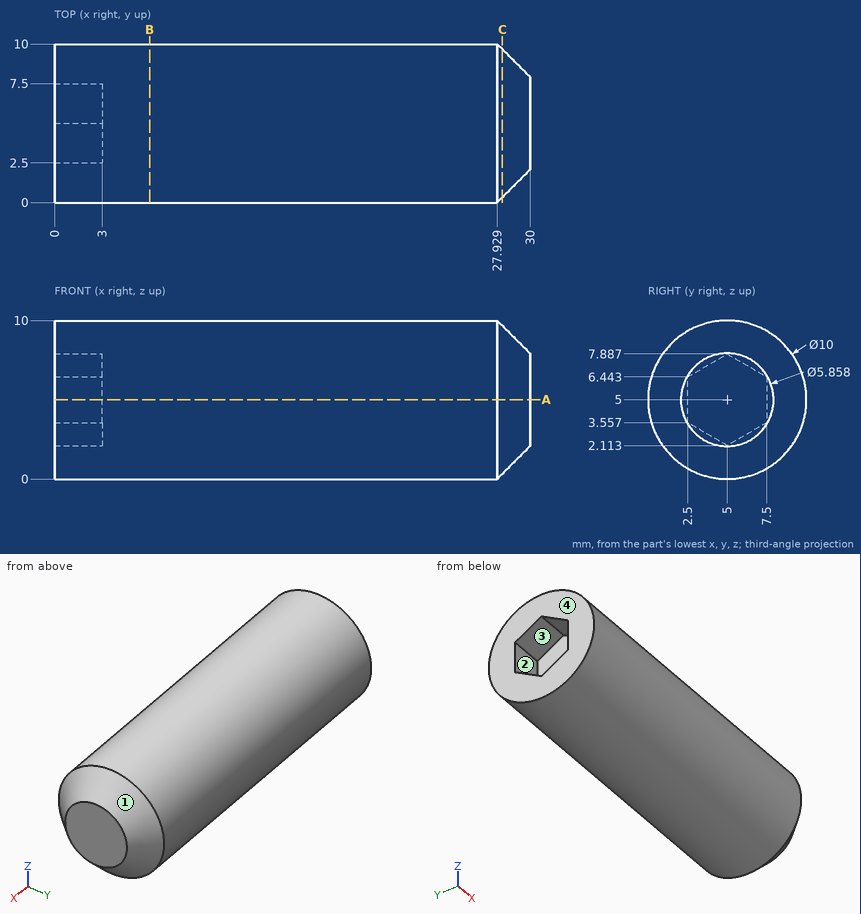
Study the drawing (mm; zero at the part's minimum x, y, z) and answer. Coordinates: 2 decimals unless noted, no trailing zeros. Order: outer loops, then holes, each group sorted by start corner. A loop starts at its lowest first (then second) coordinate and runs counter-clockwise, first axis right, second up. Notation, with made-up numbers: (81.25, -19.5) -> (90.25, -19.5) arc R19 cw to (90.25, 10.5) -> close; hole circle Ø6 at (-0.5, 79.5). An arc over 180 degrees is marked (long way). Answer in a Markdown table with one row per item. Add a question column.
Item 1: Find the intervals of material crossed by L1, parallel to Z at x = 9.25, y = 5.25; L2, parallel to X at y = 4.25, z = 5.5; L3, parallel to Y at x = 2.25, z = 4.5 (1 decimal), in increasing order. Write a range as from..to.
Item 2: Find section A-A (z = 5). Write down the section's boundary in (x, y).
Item 3: Each of these flat-tipped pins is pushed along its axis until it touches: P1, Ø3, axis at x = 23.5, z = 7, coming from the -Y side (1 decimal); P2, Ø3, axis at x = 21, y = 2.5, coming from the -Z side; P3, Ø1, axis at x = 26.5, y = 3, coming from the -Z side. Where does it stop, or does it pass through?
Item 4: Find section B-B (x = 6). Write down the section's boundary in (y, z).
Item 5: Find section C-C (x = 28.25). Write down the section's boundary in (y, z), then the cut area to 3 significant figures.
Item 6: Determine the mould class of the marked faces 1, 2, 3 and 4 for opening direction Z: +Z half, -Z half, draft (parallel to the pull), parting line (faces both ways), or undercut.
Result set:
| question | item | result |
|---|---|---|
| 1 | L1 | z = 0.01..9.99 |
| 1 | L2 | x = 3..30 |
| 1 | L3 | y = 0..2.5, 7.5..10 |
| 2 | outline | (0, 0) -> (27.93, 0) -> (30, 2.07) -> (30, 7.93) -> (27.93, 10) -> (0, 10) -> (0, 7.5) -> (3, 7.5) -> (3, 2.5) -> (0, 2.5) -> close |
| 3 | P1 | stops at y = 0 |
| 3 | P2 | stops at z = 0.1 |
| 3 | P3 | stops at z = 0.23 |
| 4 | outline | circle Ø10 at (5, 5) |
| 5 | outline | circle Ø9.36 at (5, 5) |
| 5 | area | 68.8 mm² |
| 6 | face 1 | parting line |
| 6 | face 2 | undercut |
| 6 | face 3 | undercut |
| 6 | face 4 | draft |
